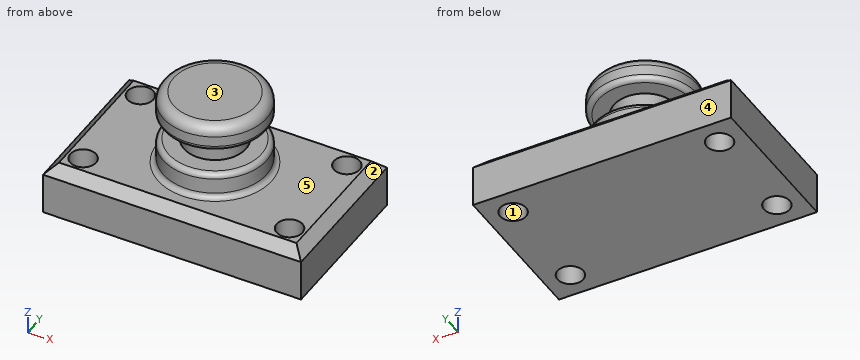
from build123d import *

# Parameters (mm, degrees)
F0_W     = 127
F0_H     = 76.2
F1_DEPTH = 25.4
F2_R     = 6.35
F3_DEPTH = 25.401
F4_W     = 25.4
F4_H     = 38.1
F6_W     = 25.4
F6_H     = 12.7
F8_SIZE  = 5.08
F9_R     = 2.54
F10_R    = 5.08


with BuildPart() as f1:
    # F0 (on Top) → F1 (new body)
    with BuildSketch(Plane.XY):
        Rectangle(F0_W, F0_H)
    extrude(amount=F1_DEPTH)

    # F2 (on face) → F3 (cut, through all)
    with BuildSketch(Plane.XY.offset(25.4)):
        with Locations((50.8, 25.4)):
            Circle(F2_R)
        with Locations((50.8, -25.4)):
            Circle(F2_R)
        with Locations((-50.8, -25.4)):
            Circle(F2_R)
        with Locations((-50.8, 25.4)):
            Circle(F2_R)
    extrude(amount=-F3_DEPTH, mode=Mode.SUBTRACT)

    # F4 (on Front) → F5 (revolve)
    with BuildSketch(Plane.XZ):
        with Locations((-12.7, 44.45)):
            Rectangle(F4_W, F4_H)
    revolve(axis=Axis((0, 0, 44.45), (0, 0, 1)))

    # F6 (on Front) → F7 (revolve, cut)
    with BuildSketch(Plane.XZ):
        with Locations((-27.94, 44.45)):
            Rectangle(F6_W, F6_H)
    revolve(axis=Axis((0, 0, 63.5), (0, 0, -1)), mode=Mode.SUBTRACT)

    # F8
    f8_edges = [f1.edges().sort_by_distance(p)[0] for p in [
        (63.5, 0, 25.4),
        (0, 38.1, 25.4),
        (-63.5, 0, 25.4),
        (0, -38.1, 25.4),
    ]]
    chamfer(f8_edges, length=F8_SIZE)

    # F9
    f9_edges = [f1.edges().sort_by_distance(p)[0] for p in [
        (25.4, 0, 38.1),
        (25.4, 0, 25.4),
        (25.4, 0, 50.8),
    ]]
    fillet(f9_edges, radius=F9_R)

    # F10
    f10_edges = [f1.edges().sort_by_distance(p)[0] for p in [
        (25.4, 0, 63.5),
    ]]
    fillet(f10_edges, radius=F10_R)


solid = f1.part
Source: CAD feature listing. Evaluate the final solid. Frame: model axes, mm. Face numbers are marked on the shaded views. A direction names the side the tool comes from. Coordinates: 2 decimals unless noted, no trailing zeros. Loops run counter-clockwise (first coordinate to the right, second up) from the corner with the lowest first, then second, coordinate; pieces in that order, holes last. Notation, with made-up numbers: (-25, 56.5) - (32, 56.5) arc R12 cw to (32, 72.5) - close; hole circle Ø6 at (-35.75, -35.75). An arc over 180 degrees is marked (long way). One line per question, with ' | ' between items.
1) Section C-C, the plane y = 0. Return loops of the section in (x, z), then the cut area to 3 significant figures.
Report:
outline: (-63.5, 0) - (63.5, 0) - (63.5, 20.32) - (58.42, 25.4) - (27.94, 25.4) arc R2.54 cw to (25.4, 27.94) - (25.4, 35.56) arc R2.54 ccw to (22.86, 38.1) - (15.24, 38.1) - (15.24, 50.8) - (22.86, 50.8) arc R2.54 ccw to (25.4, 53.34) - (25.4, 58.42) arc R5.08 ccw to (20.32, 63.5) - (-20.32, 63.5) arc R5.08 ccw to (-25.4, 58.42) - (-25.4, 53.34) arc R2.54 ccw to (-22.86, 50.8) - (-15.24, 50.8) - (-15.24, 38.1) - (-22.86, 38.1) arc R2.54 ccw to (-25.4, 35.56) - (-25.4, 27.94) arc R2.54 cw to (-27.94, 25.4) - (-58.42, 25.4) - (-63.5, 20.32) - close | area: 4,860 mm²
2) Section A-A, the plane x = -50.8. Return loops of the section in (y, z).
Report:
outline: (-38.1, 0) - (-31.75, 0) - (-31.75, 25.4) - (-33.02, 25.4) - (-38.1, 20.32) - close; (-19.05, 0) - (19.05, 0) - (19.05, 25.4) - (-19.05, 25.4) - close; (31.75, 0) - (38.1, 0) - (38.1, 20.32) - (33.02, 25.4) - (31.75, 25.4) - close
3) Line query: line 1 along Y through (x, z) = (-50.8, 7.75); line 2 along X through (y, z) = (25, 8); line 3 along Y through (x, z) = (-45, 9). Output: solid intervals per line, ascending.
Report:
line 1: y = -38.1 to -31.75, -19.05 to 19.05, 31.75 to 38.1 | line 2: x = -63.5 to -57.14, -44.46 to 44.46, 57.14 to 63.5 | line 3: y = -38.1 to -27.99, -22.81 to 22.81, 27.99 to 38.1
4) Set-up query: the marked faces 4 and 5. Return all of +Z, -Z, +X, -X, +Y, -Y with unobstructed straight access to the full face (end or side cutting, diameter ignored); none if empty.
Report:
face 4: +Z, -Z, +X, -X, +Y | face 5: +Z
5) Section D-D, the plane x = 0. Return loops of the section in (y, z).
Report:
outline: (-38.1, 0) - (38.1, 0) - (38.1, 20.32) - (33.02, 25.4) - (27.94, 25.4) arc R2.54 cw to (25.4, 27.94) - (25.4, 35.56) arc R2.54 ccw to (22.86, 38.1) - (15.24, 38.1) - (15.24, 50.8) - (22.86, 50.8) arc R2.54 ccw to (25.4, 53.34) - (25.4, 58.42) arc R5.08 ccw to (20.32, 63.5) - (-20.32, 63.5) arc R5.08 ccw to (-25.4, 58.42) - (-25.4, 53.34) arc R2.54 ccw to (-22.86, 50.8) - (-15.24, 50.8) - (-15.24, 38.1) - (-22.86, 38.1) arc R2.54 ccw to (-25.4, 35.56) - (-25.4, 27.94) arc R2.54 cw to (-27.94, 25.4) - (-33.02, 25.4) - (-38.1, 20.32) - close
6) Section B-B, the plane z = 9. Return loops of the section in (x, y).
Report:
outline: (-63.5, -38.1) - (63.5, -38.1) - (63.5, 38.1) - (-63.5, 38.1) - close; hole circle Ø12.7 at (-50.8, -25.4); hole circle Ø12.7 at (-50.8, 25.4); hole circle Ø12.7 at (50.8, -25.4); hole circle Ø12.7 at (50.8, 25.4)
7) First-contact query: P1, Ø1.5, axis at y = -15, z = 24.5, coming from the +X side; P2, Ø8, axis at x = 45, y = -26, coming from the +Z side; P3, Ø12, axis at y = -10.5, z = 42, coming from the -X side. Flat tips, straight axial feed; report the tip coordinate or a pass-through.
Report:
P1: stops at x = 60.07 | P2: stops at z = 25.4 | P3: stops at x = -23.93
8) Pull-direction query (X, two-part tool) for the marked faces 1, 2 and 3; classes: released by +X, released by -X, zero draft, split by the parting line, or undercut.
Report:
face 1: undercut | face 2: released by +X | face 3: zero draft
